from build123d import *

# Parameters (mm, degrees)
SKETCH1_R                 = 55.2
BOSS_EXTRUDE1_DEPTH       = 3
SKETCH2_R                 = 55
CUT_EXTRUDE1_DEPTH        = 79.12221195
SKETCH4_R                 = 55.2
BOSS_EXTRUDE2_DEPTH       = 18.5
BOSS_EXTRUDE4_DEPTH       = 3
SKETCH6_R                 = 9.5
SKETCH6_W                 = 16
SKETCH6_H                 = 30
BOSS_EXTRUDE3_DEPTH       = 3
BOSS_EXTRUDE9_REACH       = 83.176
SKETCH15_R                = 3
F_3_0MM_DOWEL_HOLE2_D     = 3
F_3_0MM_DOWEL_HOLE2_DEPTH = 14
F_3_0MM_DOWEL_HOLE2_TIP   = 0.901290929


with BuildPart() as part:
    # Sketch1 → Boss-Extrude1 (new body)
    with BuildSketch(Plane(origin=(0, 0, 0), x_dir=(1, 0, 0), z_dir=(0, 1, 0))):
        with Locations(Location((0, 0, 0), (0, 0, 270))):
            Circle(SKETCH1_R)
    extrude(amount=BOSS_EXTRUDE1_DEPTH)

    # Sketch2 → Cut-Extrude1 (cut, through all)
    with BuildSketch(Plane(origin=(0, 3, 0), x_dir=(1, 0, 0), z_dir=(0, 1, 0))):
        with Locations(Location((0, 0, 0), (0, 0, 270))):
            Circle(SKETCH2_R)
    extrude(amount=-CUT_EXTRUDE1_DEPTH, mode=Mode.SUBTRACT)

    # Sketch4 → Boss-Extrude2 (add)
    with BuildSketch(Plane(origin=(0, 3, 0), x_dir=(1, 0, 0), z_dir=(0, 1, 0))):
        with Locations(Location((0, 0, 0), (0, 0, 270))):
            Circle(SKETCH4_R)
        with BuildLine():
            Line((-45.2, -5), (-45.2, 5))
            Line((-45.2, 5), (-53.768020235, 5))
            ThreePointArc((-53.768020235, 5), (54, 0), (-53.768020235, -5))
            Line((-53.768020235, -5), (-45.2, -5))
        make_face(mode=Mode.SUBTRACT)
    extrude(amount=BOSS_EXTRUDE2_DEPTH)

    # Sketch8 → Boss-Extrude4 (add)
    with BuildSketch(Plane.XZ.offset(-3)):
        with BuildLine():
            Line((-45.2, 5), (-54.772255751, 5))
            ThreePointArc((-54.772255751, 5), (-55, 0), (-54.772255751, -5))
            Line((-54.772255751, -5), (-45.2, -5))
            Line((-45.2, -5), (-45.2, 5))
        make_face()
    extrude(amount=BOSS_EXTRUDE4_DEPTH)

    # Sketch6 → Boss-Extrude3 (add)
    with BuildSketch(Plane(origin=(0, 21.5, 0), x_dir=(1, 0, 0), z_dir=(0, 1, 0))):
        with BuildLine():
            Line((-55.274315916, -5), (-54.973084323, -5))
            ThreePointArc((-54.973084323, -5), (0, -55.2), (54.973084323, -5))
            Line((54.973084323, -5), (55.274315916, -5))
            ThreePointArc((55.274315916, -5), (55.5, 0), (55.274315916, 5))
            Line((55.274315916, 5), (54.973084323, 5))
            ThreePointArc((54.973084323, 5), (0, 55.2), (-54.973084323, 5))
            Line((-54.973084323, 5), (-55.274315916, 5))
            ThreePointArc((-55.274315916, 5), (-55.5, 0), (-55.274315916, -5))
        make_face()
        with Locations(Location((-22.20107336, 19.059873591, 0), (0, 0, 270))):
            Circle(SKETCH6_R, mode=Mode.SUBTRACT)
        with Locations((19.213108786, 13)):
            Rectangle(SKETCH6_W, SKETCH6_H, mode=Mode.SUBTRACT)
    extrude(amount=BOSS_EXTRUDE3_DEPTH)

    # Sketch15 → Boss-Extrude9 (add, up to next)
    with BuildSketch(Plane.XZ.offset(-3), mode=Mode.PRIVATE) as boss_extrude9_sk1:
        with Locations(Location((0, 42, 0), (0, 0, 270))):
            Circle(SKETCH15_R)
    boss_extrude9_tool1 = extrude(boss_extrude9_sk1.sketch, amount=-BOSS_EXTRUDE9_REACH, mode=Mode.PRIVATE) - part.part
    # Sketch15 → Boss-Extrude9 (add, up to next)
    with BuildSketch(Plane.XZ.offset(-3), mode=Mode.PRIVATE) as boss_extrude9_sk2:
        with Locations(Location((0, -37, 0), (0, 0, 90))):
            Circle(SKETCH15_R)
    boss_extrude9_tool2 = extrude(boss_extrude9_sk2.sketch, amount=-BOSS_EXTRUDE9_REACH, mode=Mode.PRIVATE) - part.part
    add(boss_extrude9_tool1.solids().sort_by_distance((0, 3, 42))[0])
    add(boss_extrude9_tool2.solids().sort_by_distance((0, 3, -37))[0])

    # Ø3.0mm Dowel Hole2
    with Locations(Plane(origin=(0, 3, 42), x_dir=(0, 0, -1), z_dir=(0, -1, 0))):
        with Locations((0, 0), (79, 0)):
            Hole(F_3_0MM_DOWEL_HOLE2_D / 2, depth=F_3_0MM_DOWEL_HOLE2_DEPTH)
            with Locations((0, 0, -(F_3_0MM_DOWEL_HOLE2_DEPTH + F_3_0MM_DOWEL_HOLE2_TIP / 2))):  # 118° drill point
                Cone(0, F_3_0MM_DOWEL_HOLE2_D / 2, F_3_0MM_DOWEL_HOLE2_TIP, mode=Mode.SUBTRACT)


solid = part.part
Geometry check sheet. Reference: the model listing, model coordinates, mm. A direction names the side the tool comes from. Round coordinates to 2 decimals unless told otherwise and drop trailing zeros. Order: outer loops, then holes, each group sorted by start corner. A loop starts at its lowest first (then second) coordinate and runs counter-clockwise, first axis right, second up. Notation, with made-up numbers: (74.5, 55.5) -> (94.5, 55.5) arc R24 ccw to (94.5, 74.5) -> close; hole circle Ø8 at (14, 22). An arc over 180 degrees is marked (long way). Use one line per item in the form item = value.
1. Set-up check for faces 5 (the face through (-50, 11, 5)), 6 (the face through (19, 23, -28)): record each of +Z, -Z, +X, -X, +Y, -Y from which the full face is reachable in a straight line by a thin tool's end or side.
Working result:
face_5 = -Y
face_6 = +Y, -Y
2. Mould release check, pull along X, two halves, no side actions. Record for faces 1 (the face through (-55.5, 23, -0.1)), 2 (the face through (-1.3, 3, 40.7)), 3 (the face through (-0.9, 10.1, -38.2)), 4 (the face through (-1, 24.5, -1)): pulls with the +X half, pulls with the -X half, needs draft (parallel to the pull), parting line crosses it, or undercut.
Working result:
face_1 = pulls with the -X half
face_2 = undercut
face_3 = undercut
face_4 = needs draft
3. Cross-section at D-D, the plane z = -12. Enter the section's corners in (x, y).
Working result:
outline = (-53.88, 0) -> (-53.67, 0) -> (-53.67, 3) -> (-52.65, 3) -> (-52.65, 21.5) -> (-28.56, 21.5) -> (-28.56, 24.5) -> (-53.88, 24.5) -> close; (-15.84, 21.5) -> (11.21, 21.5) -> (11.21, 24.5) -> (-15.84, 24.5) -> close; (27.21, 21.5) -> (52.65, 21.5) -> (52.65, 3) -> (53.67, 3) -> (53.67, 0) -> (53.88, 0) -> (53.88, 24.5) -> (27.21, 24.5) -> close
4. Cross-section at A-A, the plane y = 9.25. Enter the section's corners in (x, z), plus the area to 3 significant figures.
Working result:
outline = circle Ø110.4 at (0, 0); circle Ø6 at (0, -37); circle Ø6 at (0, 42); hole (-53.77, -5) arc R54 ccw (long way) to (-53.77, 5) -> (-45.2, 5) -> (-45.2, -5) -> close; hole circle Ø3 at (0, -37); hole circle Ø3 at (0, 42)
area = 541 mm^2
5. Cross-section at B-B, the plane z = 0. Enter the section's corners in (x, y).
Working result:
outline = (-55.5, 21.5) -> (-55.2, 21.5) -> (-55.2, 0) -> (-45.2, 0) -> (-45.2, 21.5) -> (11.21, 21.5) -> (11.21, 24.5) -> (-55.5, 24.5) -> close; (27.21, 21.5) -> (54, 21.5) -> (54, 3) -> (55, 3) -> (55, 0) -> (55.2, 0) -> (55.2, 21.5) -> (55.5, 21.5) -> (55.5, 24.5) -> (27.21, 24.5) -> close
6. Cross-section at C-C, the plane x = 19. Enter the section's corners in (y, z).
Working result:
outline = (0, -51.83) -> (24.5, -51.83) -> (24.5, -28) -> (21.5, -28) -> (21.5, -50.55) -> (3, -50.55) -> (3, -51.61) -> (0, -51.61) -> close; (0, 51.61) -> (3, 51.61) -> (3, 50.55) -> (21.5, 50.55) -> (21.5, 2) -> (24.5, 2) -> (24.5, 51.83) -> (0, 51.83) -> close
7. Go/stop test with flat-tipped pins: pin 1 (11 mm diameter, centred on y = 14.5, z = -1.5, fed in from +X); pin 2 (3.5 mm diameter, centred on y = 22.5, z = -15.5, fed in from -X); pin 3 (1.5 mm diameter, centred on x = 22.5, y = 23.5, fed in from -Z). Record where each tip stops, or that it passes through.
Working result:
pin_1 = 55.2
pin_2 = -53.46
pin_3 = -50.73
8. Scan lines: line 1 along X through (y, z) = (2.4, 0); line 2 along X through (y, z) = (18.5, -0.5); line 3 along X through (y, z) = (17.25, -37.5). Record each from-to range of solid material in increasing order. Write a range as from..to.
Working result:
line_1 = -55.2..-45.2, 55..55.2
line_2 = -55.2..-45.2, 54..55.2
line_3 = -40.51..-38.86, -2.96..-0.96, 0.96..2.96, 38.86..40.51
